Source: CAD feature listing. Evaluate the final solid. Frame: model axes, mm. Face numbers are marked on the shaded views. A direction names the side the tool comes from. Give positions to 0.01 mm unless a question says otherwise; leave off trailing zeros. Loops run counter-clockwise (first coordinate to the right, second up) from the corner with the lowest first, then second, coordinate; pieces in that order, holes last. Notation, with made-up numbers: M 81.5,81 L 104.5,81 A25 ccw 104.5,93 Z; hole C -33,89.5 d2. An arc over 180 degrees is marked long. Put each result on its own line as item: value. Start each with the question number.
```python
from build123d import *

# Parameters (mm, degrees)
SKETCH1_R                                  = 25
BOSS_EXTRUDE1_DEPTH                        = 13
SKETCH3_W                                  = 22
SKETCH3_H                                  = 50
SKETCH3_H_2                                = 30
CUT_EXTRUDE1_DEPTH                         = 10
CUT_EXTRUDE2_DEPTH                         = 38.669616404
CUT_EXTRUDE2_DEPTH_BACK                    = 38.669616404
SKETCH4_R                                  = 1.75
SKETCH5_R                                  = 1.75
CUT_EXTRUDE3_DEPTH                         = 37.742346142
MIRROR1_AT_THE_SECOND_PLANE_COPY_1_SKETC_R = 1.75
MIRROR1_AT_THE_SECOND_PLANE_COPY_1_DEPTH   = 37.742346142


with BuildPart() as part:
    # Sketch1 → Boss-Extrude1 (new body)
    with BuildSketch(Plane.XY):
        with Locations(Location((0, 0, 0), (0, 0, 180))):
            Circle(SKETCH1_R)
    extrude(amount=BOSS_EXTRUDE1_DEPTH)

    # Sketch3 → Cut-Extrude1 (cut)
    with BuildSketch(Plane.XY.offset(13)):
        Rectangle(SKETCH3_W, SKETCH3_H)
        with Locations((25, 0)):
            Rectangle(SKETCH3_W, SKETCH3_H_2)
        with Locations((-25, 0)):
            Rectangle(SKETCH3_W, SKETCH3_H_2)
    extrude(amount=-CUT_EXTRUDE1_DEPTH, mode=Mode.SUBTRACT)

    # Sketch4 → Cut-Extrude2 (cut, two sides: drawn at the far end of the back side and taken through both)
    with BuildSketch(Plane(origin=(0, 0, 0), x_dir=(0, 0, -1), z_dir=(1, 0, 0)).offset(-CUT_EXTRUDE2_DEPTH_BACK)):
        with Locations((-9, 7.5)):
            Circle(SKETCH4_R)
        with Locations((-9, 0)):
            Circle(SKETCH4_R)
        with Locations((-9, -7.5)):
            Circle(SKETCH4_R)
    extrude(amount=CUT_EXTRUDE2_DEPTH + CUT_EXTRUDE2_DEPTH_BACK, mode=Mode.SUBTRACT)

    # Sketch5 → Cut-Extrude3 (cut, through all)
    with BuildSketch(Plane.XY.offset(3)):
        with Locations((-19, 5)):
            Circle(SKETCH5_R)
        with Locations((-5, 19)):
            Circle(SKETCH5_R)
    cut_extrude3 = extrude(amount=-CUT_EXTRUDE3_DEPTH, mode=Mode.SUBTRACT)

    # Mirror1: Cut-Extrude3 across plane
    add(cut_extrude3.mirror(Plane(origin=(0, 0, 0), x_dir=(0, 0, 1), z_dir=(1, 0, 0))), mode=Mode.SUBTRACT)

    # Mirror1 at the second plane: Cut-Extrude3 across plane
    add(cut_extrude3.mirror(Plane.ZX), mode=Mode.SUBTRACT)

    # Mirror1 at the second plane copy 1 sketc → Mirror1 at the second plane copy 1 (cut, through all)
    with BuildSketch(Plane(origin=(0, 0, 3), x_dir=(-1, 0, 0), z_dir=(0, 0, 1))):
        with Locations((-19, 5)):
            Circle(MIRROR1_AT_THE_SECOND_PLANE_COPY_1_SKETC_R)
        with Locations((-5, 19)):
            Circle(MIRROR1_AT_THE_SECOND_PLANE_COPY_1_SKETC_R)
    extrude(amount=-MIRROR1_AT_THE_SECOND_PLANE_COPY_1_DEPTH, mode=Mode.SUBTRACT)


solid = part.part
```
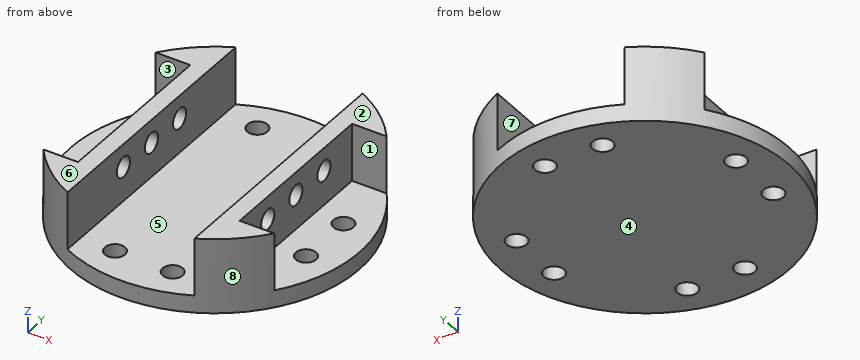
1. Pull-direction query (X, two-part tool) for the marked faces 6, 7 and 8; classes: released by +X, released by -X, zero draft, split by the parting line, or undercut.
2. Set-up query: the marked faces 1, 2, 3, 4 and 5. Return all of +Z, -Z, +X, -X, +Y, -Y with unobstructed straight access to the full face (end or side cutting, diameter ignored); none if empty.
3. Contact query for flat-ended pins moving along their axis: pin 1 (4 mm diameter, centred on x = -19, y = 5, fed in from +Z); pin 2 (10 mm diameter, centred on x = 8.5, y = 13, fed in from -Z); pin 3 (1.5 mm diameter, centred on x = 4.5, z = 3, fed in from -Y); pin 4 (2 mm diameter, centred on x = -17, z = 5, fed in from -Y). Output: stop coordinate, or through.
4. Section A-A, the plane z = 6.5. Output: boundary loops of the cut face in (x, y), plus the area to 3 significant figures.
5. Ray query, line 1 (X direction, y = -9.5, z = 6.5); line 2 (Y direction, x = 5, z = 0.9); line 3 (Z direction, x = 13.4, y = 0). Return the intervals inside material, ascending.
6. Section D-D, the plane x = -19. Output: boundary loops of the cut face in (y, z).
7. Section C-C, the plane y = -5. Output: boundary loops of the cut face in (x, z).
8. Section B-B, the plane z = 2. State how many separate pieces and enclosed holes the cut face has, plus the area to 3 significant figures.
Results found:
1. face 6: zero draft
1. face 7: undercut
1. face 8: split by the parting line
2. face 1: +Z, +X
2. face 2: +Z, +X, -X, +Y, -Y
2. face 3: +Z, -X
2. face 4: -Z, +X, -X, +Y, -Y
2. face 5: +Z, +Y, -Y
3. pin 1: z = 3
3. pin 2: z = 0
3. pin 3: y = -24.72
3. pin 4: y = -19.21
4. outline: M -20,-15 A25 ccw -11,-22.45 L -11,22.45 A25 ccw -20,15 L -14,15 L -14,-15 Z; M 11,-22.45 A25 ccw 20,-15 L 14,-15 L 14,15 L 20,15 A25 ccw 11,22.45 Z
4. area: 336 mm²
5. line 1: -14 to -11, 11 to 14
5. line 2: -24.49 to -20.75, -17.25 to 17.25, 20.75 to 24.49
5. line 3: 0 to 7.25, 10.75 to 13
6. outline: M -16.25,0 L -6.75,0 L -6.75,3 L -15,3 L -15,13 L -16.25,13 Z; M -3.25,0 L 3.25,0 L 3.25,3 L -3.25,3 Z; M 6.75,0 L 16.25,0 L 16.25,13 L 15,13 L 15,3 L 6.75,3 Z
7. outline: M -24.49,0 L -20.75,0 L -20.75,3 L -24.49,3 Z; M -17.25,0 L 17.25,0 L 17.25,3 L 14,3 L 14,13 L 11,13 L 11,3 L -11,3 L -11,13 L -14,13 L -14,3 L -17.25,3 Z; M 20.75,0 L 24.49,0 L 24.49,3 L 20.75,3 Z
8. separate pieces: 1
8. enclosed holes: 8
8. area: 1,890 mm²
